Model file for the job. Use its own axes, mm. Give positions to 0.01 mm unless a question says otherwise; leave off trailing zeros. Write each loop counter-clockwise with the first axis right and the second up, starting at its lowest first coordinate (ties: lowest second). Pieces come first, ordered by that corner, then holes. Notation, with made-up numbers: (22, 89.25) - (49, 89.25) arc R11 ccw to (49, 108.25) - close; hole circle Ø2 at (-34.5, -14). An arc over 180 degrees is marked (long way). One line per item, written item: value. Start each with the question number.
(1) Probe L1, parallel to X at y = -7.25, z = 440; L2, parallel to Y at x = 0.75, z = 430; L3, parallel to Y at x = 5.35, z = 508. List the from-to ranges inside material, lowest first.
(2) Drop flat-ended pins along their axis: P1, Ø3, axis at x = 2.5, y = -7, coming from the +Z side; P2, Ø5, axis at x = 0, z = 12.7, coming from the -Y side; P3, Ø5, axis at x = 4, y = 9.5, coming from the -Z side. Give the stop position or say it passes through.
(3) Cut at A-A, the plane z = 427. List the corners of the cut face in (x, y).
from build123d import *

# Parameters (mm, degrees)
SKETCH1_W           = 12.7
SKETCH1_H           = 25.4
SKETCH1_W_2         = 9.525
SKETCH1_H_2         = 22.225
BOSS_EXTRUDE1_DEPTH = 546.1
SKETCH2_R           = 3.81
SKETCH2_R_2         = 2.75
CUT_EXTRUDE1_DEPTH  = 547.395269013
CUT_EXTRUDE3_REACH  = 548.395
CUT_EXTRUDE5_REACH  = 548.727
SKETCH5_R           = 2.75


with BuildPart() as part:
    # Sketch1 → Boss-Extrude1 (new body)
    with BuildSketch(Plane.XY):
        Rectangle(SKETCH1_W, SKETCH1_H)
        Rectangle(SKETCH1_W_2, SKETCH1_H_2, mode=Mode.SUBTRACT)
    extrude(amount=BOSS_EXTRUDE1_DEPTH)

    # Sketch2 → Cut-Extrude1 (cut, through all)
    with BuildSketch(Plane(origin=(6.35, 0, 0), x_dir=(0, 0, -1), z_dir=(1, 0, 0))):
        with Locations((-508, 0)):
            Circle(SKETCH2_R)
        with Locations((-520.7, 0)):
            Circle(SKETCH2_R_2)
        with Locations((-495.3, 0)):
            Circle(SKETCH2_R_2)
        with BuildLine():
            Line((-31.75, -3.302), (-44.45, -3.302))
            ThreePointArc((-44.45, -3.302), (-47.752, 0), (-44.45, 3.302))
            Line((-44.45, 3.302), (-31.75, 3.302))
            ThreePointArc((-31.75, 3.302), (-28.448, 0), (-31.75, -3.302))
        make_face()
    extrude(amount=-CUT_EXTRUDE1_DEPTH, mode=Mode.SUBTRACT)

    # Sketch4 → Cut-Extrude3 (cut, up to next)
    with BuildSketch(Plane.ZY.offset(6.35), mode=Mode.PRIVATE) as cut_extrude3_sk1:
        with BuildLine():
            Line((35.56, 5), (66.04, 5))
            ThreePointArc((66.04, 5), (71.04, 0), (66.04, -5))
            Line((66.04, -5), (35.56, -5))
            ThreePointArc((35.56, -5), (30.56, 0), (35.56, 5))
        make_face()
    cut_extrude3_tool1 = extrude(cut_extrude3_sk1.sketch, amount=-CUT_EXTRUDE3_REACH, mode=Mode.PRIVATE) & part.part
    # Sketch4 → Cut-Extrude3 (cut, up to next)
    with BuildSketch(Plane.ZY.offset(6.35), mode=Mode.PRIVATE) as cut_extrude3_sk2:
        with BuildLine():
            Line((495.3, 5), (520.7, 5))
            ThreePointArc((520.7, 5), (525.7, 0), (520.7, -5))
            Line((520.7, -5), (495.3, -5))
            ThreePointArc((495.3, -5), (490.3, 0), (495.3, 5))
        make_face()
    cut_extrude3_tool2 = extrude(cut_extrude3_sk2.sketch, amount=-CUT_EXTRUDE3_REACH, mode=Mode.PRIVATE) & part.part
    add(cut_extrude3_tool1.solids().sort_by_distance((-6.35, 0, 50.8))[0], mode=Mode.SUBTRACT)
    add(cut_extrude3_tool2.solids().sort_by_distance((-6.35, 0, 508))[0], mode=Mode.SUBTRACT)

    # Sketch5 → Cut-Extrude5 (cut, up to next)
    with BuildSketch(Plane.XZ.offset(12.7), mode=Mode.PRIVATE) as cut_extrude5_sk1:
        with Locations(Location((0, 533.4, 0), (0, 0, 270))):
            Circle(SKETCH5_R)
    cut_extrude5_tool1 = extrude(cut_extrude5_sk1.sketch, amount=-CUT_EXTRUDE5_REACH, mode=Mode.PRIVATE) & part.part
    # Sketch5 → Cut-Extrude5 (cut, up to next)
    with BuildSketch(Plane.XZ.offset(12.7), mode=Mode.PRIVATE) as cut_extrude5_sk2:
        with Locations(Location((0, 12.7, 0), (0, 0, 270))):
            Circle(SKETCH5_R)
    cut_extrude5_tool2 = extrude(cut_extrude5_sk2.sketch, amount=-CUT_EXTRUDE5_REACH, mode=Mode.PRIVATE) & part.part
    add(cut_extrude5_tool1.solids().sort_by_distance((0, -12.7, 533.4))[0], mode=Mode.SUBTRACT)
    add(cut_extrude5_tool2.solids().sort_by_distance((0, -12.7, 12.7))[0], mode=Mode.SUBTRACT)


solid = part.part
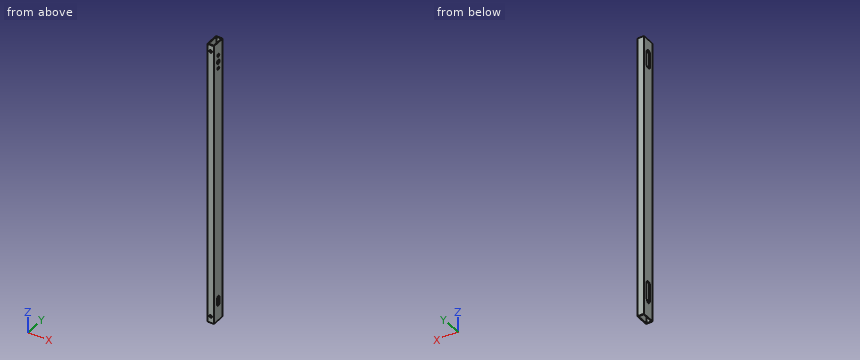
Answers follow:
1. L1: x = -6.35 to -4.76, 4.76 to 6.35
1. L2: y = -12.7 to -11.11, 11.11 to 12.7
1. L3: y = -12.7 to -3.81, 3.81 to 12.7
2. P1: passes through
2. P2: stops at y = 11.11
2. P3: stops at z = 0
3. outline: (-6.35, -12.7) - (6.35, -12.7) - (6.35, 12.7) - (-6.35, 12.7) - close; hole (-4.76, -11.11) - (4.76, -11.11) - (4.76, 11.11) - (-4.76, 11.11) - close
